Design review of the part built by this model. Coordinates are the model's own, in mm. Face numbers are marked on the shaded views. Round coordinates to 2 decimals unless told otherwise and drop trailing zeros. Loops run counter-clockwise (first coordinate to the right, second up) from the corner with the lowest first, then second, coordinate; pieces in that order, holes last. Notation, with made-up numbers: M 34,65.5 L 41,65.5 A27 ccw 41,87.5 Z; hole C 10,65 d6. An arc over 180 degrees is marked long. Use a Markdown table: item, result.
Autodesk Inventor part; units mm, degrees
ref_plane "YZ Plane" through (0, 0, 0) normal (1, 0, 0) x (0, 1, 0)
ref_plane "XZ Plane" through (0, 0, 0) normal (0, 1, 0) x (-1, 0, 0)
ref_plane "XY Plane" through (0, 0, 0) normal (0, 0, 1) x (1, 0, 0)
sketch "Basisskizze" plane through (0, 0, 0) normal (0, 1, 0) x (-1, 0, 0)
  line L0 (0, -56) -> (0, 56) construction
  line L1 (56, 0) -> (-56, 0) construction
  line L2 (40, -40) -> (-40, -40)
  line L3 (-40, -40) -> (-40, 40)
  line L4 (-40, 40) -> (40, 40)
  line L5 (40, 40) -> (40, -40)
  line L6 (10, -40) -> (10, 10) construction
  line L7 (10, 10) -> (-40, 10) construction
  point P0 (0, 0)
  dimension "d2" = 80
  dimension "d3" = 30
  dimension "d4" = 30
extrude "Grundkörper" add sketch "Basisskizze" along normal mid plane 20
sketch "Skizze5" plane through (0, -10, 0) normal (0, -1, 0) x (1, 0, 0)
  line L0 (-10, -40) -> (40, 10)
  line L1 (40, 40) -> (-40, 40)
  line L2 (-40, 40) -> (-40, -40)
  line L3 (-40, -40) -> (40, -40)
  line L4 (40, -40) -> (40, 40)
  point P0 (0, 0)
  dimension "d19" = 30
  dimension "d20" = 30
extrude "Abschnitt" cut sketch "Skizze5" against normal through all contours L0 L4 L3
sketch "Skizze6" plane through (0, -10, 0) normal (0, -1, 0) x (1, 0, 0)
  line L0 (-10, -40) -> (40, 10)
  line L1 (-40, -40) -> (-40, 40)
  line L2 (15, -15) -> (-40, 40) construction
  line L3 (-40, -40) -> (-10, -40)
  line L4 (-10, -40) -> (-10, 40)
  line L5 (-40, 40) -> (40, 40)
  line L6 (40, 10) -> (-40, 10)
  point P0 (0, 0)
  point P1 (0, 0)
  dimension "d23" = 40
  dimension "d24" = 21.2132
hole "DIN7984_M8" at (0, -10, 0) direction (0, 1, 0) diameter 9 end through all counterbore diameter 15 counterbore depth 5.4
sketch "Skizze7" plane through (0, 10, 0) normal (0, 1, 0) x (1, 0, 0)
  line L0 (40, -10) -> (-10, 40) construction
  line L1 (15, 15) -> (-40, -40) construction
  line L2 (22.0711, 7.9289) -> (-32.9289, -47.0711)
  line L3 (-32.9289, -47.0711) -> (-47.0711, -32.9289)
  line L4 (-47.0711, -32.9289) -> (7.9289, 22.0711)
  line L5 (7.9289, 22.0711) -> (22.0711, 7.9289)
  point P0 (0, 0)
  dimension "d32" = 20
extrude "NUT_Torsionssicherung" cut sketch "Skizze7" against normal blind 5
sketch "Skizze8" plane through (0, -10, 0) normal (0, -1, 0) x (1, 0, 0)
  line L0 (-10, -40) -> (-40, -40)
  line L1 (-25.8579, 40) -> (40, 40)
  line L2 (-40, 40) -> (-40, -40)
  line L3 (-40, 25.8579) -> (7.9289, -22.0711)
  line L4 (-25, -40) -> (-25, 40) construction
  line L5 (40, 40) -> (-40, 40)
  line L6 (-40, -40) -> (-10, -40)
  line L7 (40, 40) -> (40, 10)
  line L8 (40, 25) -> (-40, 25) construction
  line L9 (40, 10) -> (40, 40)
  point P0 (0, 0)
  point P1 (-25, 25)
  point P2 (-25, 0)
  point P3 (-25, -25)
  point P4 (0, 25)
  point P5 (25, 25)
  dimension "d38" = 15
  dimension "d39" = 15
  dimension "d43" = 25
  dimension "d48" = 25
  dimension "d49" = 25
hole "M8_Profilgewinde" at (-25, -10, 25) at (-25, -10, 0) at (-25, -10, -25) at (0, -10, 25) at (25, -10, 25) direction (0, 1, 0) diameter 6.647 end through all countersink diameter 8 countersink angle 90
sketch "Skizze9" plane through (0, 5, 0) normal (0, 1, 0) x (1, 0, 0)
  circle A0 centre (-25, -25) radius 3.3235 construction
  circle A1 centre (0, 0) radius 4.5 construction
  line L0 (40, -40) -> (-40, -40)
  line L1 (-40, -40) -> (0, 0) construction
  line L2 (-17.9289, -32.0711) -> (-32.0711, -17.9289) construction
  line L3 (-40, -25.8579) -> (7.9289, 22.0711)
  line L4 (22.0711, 7.9289) -> (-25.8579, -40)
  line L5 (-40, 40) -> (-40, -25.8579)
  line L6 (7.9289, 22.0711) -> (22.0711, 7.9289)
  point P0 (0, 0)
  point P1 (-12.7279, -12.7279)
  point P2 (-33.5876, -33.5876)
  dimension "d72" = 18
  dimension "d73" = 47.5
hole "M5_Bohrung" at (-12.7279, 5, 12.7279) at (-33.5876, 5, 33.5876) direction (0, -1, 0) diameter 4.134 end through all countersink diameter 5 countersink angle 90
equation "\"d4\" = d3"
properties part number "200-20-ROCKER-CONNECTOR-04" material "Aluminium 6061"
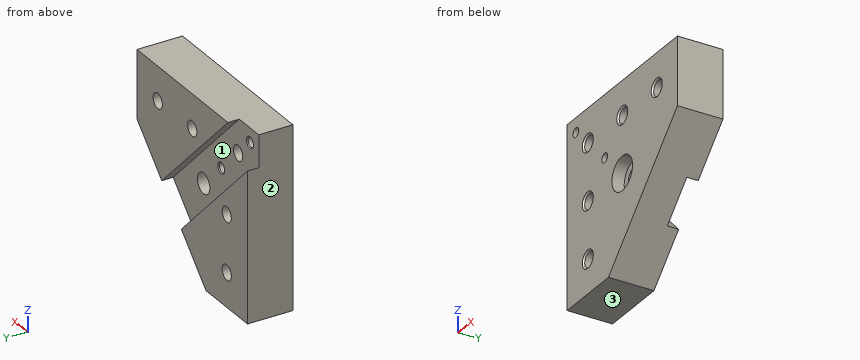
1. Take a section at B-B on x = 25. Give the boundary of the cut face in (y, z), and give its area (3 significant figures).
Check values:
| item | result |
|---|---|
| outline | M -10,-5 L 10,-5 L 10,21.68 L -9.32,21.68 L -10,21 Z; M -10,29 L -9.32,28.32 L 10,28.32 L 10,40 L -10,40 Z |
| area | 767 mm² |
2. Take a section at D-D on y = -6. Count the separate pieces of the cut face and the enclosed holes in it, and give its area (3 significant figures).
Check values:
| item | result |
|---|---|
| separate pieces | 1 |
| enclosed holes | 8 |
| area | 4,770 mm² |
3. Wall thickness on line 1 along Z through (x, y) = (-25, 2); line 2 along Z through (x, y) = (0, 0.5): over which ranges is each line inside the solid? List them lowest first. Write a range as from..to.
Check values:
| item | result |
|---|---|
| line 1 | z = -40..-28.32, -21.68..-3.32, 3.32..21.68, 28.32..40 |
| line 2 | z = -30..-4.5, 4.5..21.68, 28.32..40 |
4. Take a section at C-C on z = -25. Give the boundary of the cut face in (x, y).
Check values:
| item | result |
|---|---|
| outline | M -40,-10 L -29,-10 L -28.32,-9.32 L -28.32,10 L -40,10 Z; M -21.68,-9.32 L -21,-10 L 5,-10 L 5,10 L -21.68,10 Z |
5. Take a section at A-A on y = 7.75. Give the boundary of the cut face in (x, z).
Check values:
| item | result |
|---|---|
| outline | M -40,-40 L -10,-40 L 7.93,-22.07 L -40,25.86 Z; M -25.86,40 L 22.07,-7.93 L 40,10 L 40,40 Z; hole C -25,-25 d6.65; hole C -25,0 d6.65; hole C 0,25 d6.65; hole C 25,25 d6.65 |
6. The part is to be moulded in two halves that separate along X. For the marked faces 1, 2 and 3, say which applies: pulls with the +X half, pulls with the -X half, needs draft (parallel to the pull), parting line crosses it, or undercut.
Check values:
| item | result |
|---|---|
| face 1 | undercut |
| face 2 | pulls with the -X half |
| face 3 | needs draft |
7. Insertion check: pin 1 (12 mm diameter, centred on x = 0, z = 0, fed in from -Y); pin 2 (8 mm diameter, centred on x = 31.5, z = -5.5, fed in from -Y); pin 3 (10 mm diameter, centred on x = 15, z = -19.5, fed in from +Y). Each pin has a flat end and moves straight along its axis. Give the tip position at first contact, or say it passes through.
Check values:
| item | result |
|---|---|
| pin 1 | stops at y = -4.6 |
| pin 2 | passes through |
| pin 3 | stops at y = 5 |
